Part model, mm, in its own coordinate system. A direction names the side the tool comes from. Give positions to 0.01 mm unless a question says otherwise; leave off trailing zeros. Write each loop counter-clockwise with the first axis right and the second up, starting at its lowest first coordinate (ties: lowest second). Pieces come first, ordered by that corner, then holes. Notation, with made-up numbers: M -6,41 L 10,41 A20 cw 10,53 Z; hole C 23,31.5 d1. An arc over 180 degrees is marked long. Write item = value, one per line. Start each with the question number.
from build123d import *

# Parameters (mm, degrees)
SKETCH1_R           = 29.575
SKETCH1_R_2         = 28.575
BOSS_EXTRUDE1_DEPTH = 61.5
BOSS_EXTRUDE2_START = 2.5
BOSS_EXTRUDE2_DEPTH = 46.5
CIRPATTERN1_COUNT   = 14
SKETCH4_W           = 1.75
SKETCH4_H           = 2.5
CUT_EXTRUDE1_DEPTH  = 91.308654762
CIRPATTERN2_COUNT   = 5
SKETCH5_R           = 1
CUT_EXTRUDE2_DEPTH  = 5
CIRPATTERN3_COUNT   = 5


with BuildPart() as part:
    # Sketch1 → Boss-Extrude1 (new body)
    with BuildSketch(Plane(origin=(0, 0, 0), x_dir=(1, 0, 0), z_dir=(0, 1, 0))):
        with Locations(Location((0, 0, 0), (0, 0, 270))):
            Circle(SKETCH1_R)
        with Locations(Location((0, 0, 0), (0, 0, 270))):
            Circle(SKETCH1_R_2, mode=Mode.SUBTRACT)
    extrude(amount=BOSS_EXTRUDE1_DEPTH)

    # Sketch2 → Boss-Extrude2 (add)
    with BuildSketch(Plane(origin=(0, 4.5, 0), x_dir=(-1, 0, 0), z_dir=(0, -1, 0)).offset(BOSS_EXTRUDE2_START)):
        with BuildLine():
            Line((-5, 28.134154066), (-5, 25.325))
            Line((-5, 25.325), (5, 25.325))
            Line((5, 25.325), (5, 28.134154066))
            ThreePointArc((5, 28.134154066), (2.509698445, 28.464575154), (0, 28.575))
            ThreePointArc((0, 28.575), (-2.509698445, 28.464575154), (-5, 28.134154066))
        make_face()
    boss_extrude2 = extrude(amount=-BOSS_EXTRUDE2_DEPTH)

    # CirPattern1: Boss-Extrude2 ×14 about axis
    cirpattern1_axis = Axis((0, 0, 0), (0, 1, 0))
    for i in range(1, CIRPATTERN1_COUNT):
        add(boss_extrude2.rotate(cirpattern1_axis, i * 360 / CIRPATTERN1_COUNT))

    # Sketch4 → Cut-Extrude1 (cut, through all)
    with BuildSketch(Plane.XY.offset(29.575)):
        with Locations((-28.7, 53.25)):
            Rectangle(SKETCH4_W, SKETCH4_H)
    cut_extrude1 = extrude(amount=-CUT_EXTRUDE1_DEPTH, mode=Mode.SUBTRACT)

    # CirPattern2: Cut-Extrude1 ×5 about axis
    cirpattern2_axis = Axis((0, 0, 0), (0, 1, 0))
    for i in range(1, CIRPATTERN2_COUNT):
        add(cut_extrude1.rotate(cirpattern2_axis, i * 360 / CIRPATTERN2_COUNT), mode=Mode.SUBTRACT)

    # Sketch5 → Cut-Extrude2 (cut, symmetric)
    with BuildSketch(Plane(origin=(8.776688534, 0, 27.011869813), x_dir=(-0.9510565162951524, 0, 0.30901699437495134), z_dir=(-0.30901699437495134, 0, -0.9510565162951524))):
        with Locations(Location((0, 58, 0), (0, 0, 180))):
            Circle(SKETCH5_R)
    cut_extrude2 = extrude(amount=CUT_EXTRUDE2_DEPTH, both=True, mode=Mode.SUBTRACT)

    # CirPattern3: Cut-Extrude2 ×5 about axis
    cirpattern3_axis = Axis((0, 0, 0), (0, 1, 0))
    for i in range(1, CIRPATTERN3_COUNT):
        add(cut_extrude2.rotate(cirpattern3_axis, i * 360 / CIRPATTERN3_COUNT), mode=Mode.SUBTRACT)


solid = part.part
Q1. Slice it at A-A (z = 4.5). Give the cut face in (x, y), and give its area (3 significant figures).
Q2. Probe line 1 along Z through (x, y) = (0, 15) (3 decimals); line 2 along Z through (x, y) = (-18, 4.5); line 3 along Z through (x, y) = (7, 34). List the from-to ranges inside material, lowest first.
Q3. Slice it at D-D (x = 0). Give the cut face in (y, z) (3 decimals).
Q4. Tool access for faces 4 (the face through (-21, 2, -17)), 5 (the face through (-27.825, 53, 8)), 6 (the face through (17.765, 24.924, -20.563)): list every direction of +Z, -Z, +X, -X, +Y, -Y with a clear straight run to the whole face (end or side of a thin tool).
Q5. Slice it at B-B (x = 21.5). Give the cut face in (y, z).
Q6. Two-plate mould, pull along Y, no slides. Class faces 1 (the face through (29.06, 57.16, -0.54)), 2 (the face through (12, 48.5, 24)), 3 (the face through (-24.03, 24.92, 12.77)): +Y half, -Y half, draft (parallel to the pull), parting line (faces both ways), or undercut.
Q7. Slice it at C-C (y = 58). Give the number of separate pieces and of enclosed holes in the cut face, and give its area (3 significant figures).
Q8. Drop flat-ended pins along their axis: P1, Ø1.4, axis at y = 36, z = 26, coming from the -X side; P2, Ø13, axis at x = 24.5, z = -15.5, coming from the -Y side; P3, Ø8, axis at y = 7, z = 22, coming from the +X side; P4, Ø4, axis at x = 2.5, y = 9, coming from the -Z side. Give the stop position or say it passes through.
Working result:
q1.outline = M -29.23,0 L -28.22,0 L -28.22,2 L -24.95,2 L -24.95,48.5 L -28.22,48.5 L -28.22,52 L -29.23,52 Z; M -29.23,54.5 L -28.22,54.5 L -28.22,61.5 L -29.23,61.5 Z; M 24.95,2 L 28.22,2 L 28.22,0 L 29.23,0 L 29.23,61.5 L 28.22,61.5 L 28.22,48.5 L 24.95,48.5 Z
q1.area = 426 mm2
q2.line_1 = -29.575 to -25.325, 25.325 to 29.575
q2.line_2 = -23.47 to -22.19, -20.75 to -18.05, 18.05 to 20.75, 22.19 to 23.47
q2.line_3 = -28.73 to -27.7, -26.06 to -24.74, 24.74 to 26.06, 27.7 to 28.73
q3.outline = M 0,-29.575 L 52,-29.575 L 52,-29.257 L 54.5,-29.257 L 54.5,-29.575 L 61.5,-29.575 L 61.5,-28.575 L 48.5,-28.575 L 48.5,-25.325 L 2,-25.325 L 2,-28.575 L 0,-28.575 Z; M 0,28.575 L 2,28.575 L 2,25.325 L 48.5,25.325 L 48.5,28.575 L 61.5,28.575 L 61.5,29.575 L 54.5,29.575 L 54.5,29.257 L 52,29.257 L 52,29.575 L 0,29.575 Z
q4.face_4 = -Y
q4.face_5 = +Z, -Z, -X
q4.face_6 = +Y, -Y
q5.outline = M 0,-20.31 L 52,-20.31 L 52,-18.82 L 48.5,-18.82 L 48.5,-13.66 L 2,-13.66 L 2,-18.82 L 0,-18.82 Z; M 0,18.82 L 2,18.82 L 2,13.66 L 48.5,13.66 L 48.5,18.82 L 52,18.82 L 52,20.31 L 0,20.31 Z; M 54.5,-20.31 L 61.5,-20.31 L 61.5,-18.82 L 54.5,-18.82 Z; M 54.5,18.82 L 61.5,18.82 L 61.5,20.31 L 54.5,20.31 Z
q6.face_1 = undercut
q6.face_2 = +Y half
q6.face_3 = draft
q7.separate_pieces = 5
q7.enclosed_holes = 0
q7.area = 173 mm2
q8.P1 = -15.32
q8.P2 = 0
q8.P3 = 23.47
q8.P4 = -29.57
